Autodesk Inventor part; units mm, degrees
ref_plane "YZ Plane" through (0, 0, 0) normal (1, 0, 0) x (0, 1, 0)
ref_plane "XZ Plane" through (0, 0, 0) normal (0, 1, 0) x (-1, 0, 0)
ref_plane "XY Plane" through (0, 0, 0) normal (0, 0, 1) x (1, 0, 0)
sketch "Sketch_36" plane through (0, 0, 0) normal (0, 0, 1) x (1, 0, 0)
  line L0 (1.5, 0) -> (-1.5, 0)
  arc A0 (0, 1.6) -> (0.1, 1.5) centre (0.1, 1.6) ccw
  line L1 (0.1, 1.5) -> (2.9, 1.5)
  arc A1 (2.9, 1.5) -> (3, 1.6) centre (2.9, 1.6) ccw
  line L2 (3, 1.6) -> (3, 2.025)
  line L3 (3, 2.025) -> (1.6561, 2.025)
  arc A2 (1.3439, 2.025) -> (1.6561, 2.025) centre (1.5, 2.5) ccw
  line L4 (1.3439, 2.025) -> (0, 2.025)
  line L5 (0, 2.025) -> (0, 1.6)
revolve "Revolution1" add sketch "Sketch_36" angle 360 about axis through (1.5, 0, 0) along (1, 0, 0)
sketch "Sketch_37" plane through (0, 0, 0) normal (0, 0, 1) x (1, 0, 0)
  line L0 (1.5, 0) -> (-1.5, 0)
  line L1 (0, 3.175) -> (0, 1.925)
  line L2 (0, 1.925) -> (0.05, 1.925)
  arc A0 (0.05, 1.925) -> (0.15, 2.025) centre (0.05, 2.025) ccw
  line L3 (0.15, 2.025) -> (0.15, 3.075)
  line L4 (0.15, 3.075) -> (2.85, 3.075)
  line L5 (2.85, 3.075) -> (2.85, 2.025)
  arc A1 (2.85, 2.025) -> (2.95, 1.925) centre (2.95, 2.025) ccw
  line L6 (2.95, 1.925) -> (3, 1.925)
  line L7 (3, 1.925) -> (3, 3.175)
  line L8 (3, 3.175) -> (0, 3.175)
revolve "Revolution2" cut sketch "Sketch_37" angle 360 about axis through (1.5, 0, 0) along (1, 0, 0)
sketch "Sketch_38" plane through (0, 0, 0) normal (0, 0, 1) x (1, 0, 0)
  line L0 (50, 0) -> (-50, 0)
  line L1 (0.025, 3.175) -> (0.04, 2.8625)
  line L2 (0.04, 2.8625) -> (0.025, 2.55)
  line L3 (0.025, 2.55) -> (0.025, 1.925)
  line L4 (0.025, 1.925) -> (0.055, 1.925)
  line L5 (0.055, 1.925) -> (0.085, 2.55)
  line L6 (0.085, 2.55) -> (0.085, 2.8625)
  line L7 (0.085, 2.8625) -> (0.055, 3.175)
  line L8 (0.055, 3.175) -> (0.025, 3.175)
revolve "Revolution3" add sketch "Sketch_38" angle 360 about axis through (50, 0, 0) along (1, 0, 0)
sketch "Sketch_39" plane through (0, 0, 0) normal (0, 0, 1) x (1, 0, 0)
  line L0 (50, 0) -> (-50, 0)
  line L1 (2.915, 2.8625) -> (2.915, 2.55)
  line L2 (2.915, 2.55) -> (2.945, 1.925)
  line L3 (2.945, 1.925) -> (2.975, 1.925)
  line L4 (2.975, 1.925) -> (2.975, 2.55)
  line L5 (2.975, 2.55) -> (2.96, 2.8625)
  line L6 (2.96, 2.8625) -> (2.975, 3.175)
  line L7 (2.975, 3.175) -> (2.945, 3.175)
  line L8 (2.945, 3.175) -> (2.915, 2.8625)
revolve "Revolution4" add sketch "Sketch_39" angle 360 about axis through (50, 0, 0) along (1, 0, 0)
properties part number "W 638/3 R-2Z_PART1"
Here's how the part is built. I have some questions about the finished solid (model axes, mm). Give positions to 0.01 mm unless a question says otherwise; leave off trailing zeros. Write each loop counter-clockwise with the first axis right and the second up, starting at its lowest first coordinate (ties: lowest second). Pieces come first, ordered by that corner, then holes.
(1) Will these pins go through, and if not, where does the flat tip stop? pin 1 (3 mm diameter, centred on y = -1.5, z = -2.5, fed in from +X); pin 2 (1.5 mm diameter, centred on y = 0, z = 0.5, fed in from +X); pin 3 (1 mm diameter, centred on x = 1.5, y = 1, fed in from +Z).
Output values:
pin 1: stops at x = 3
pin 2: passes through
pin 3: stops at z = 1.96
(2) Imagine slicing it at A-A, the plane x = 0.95. Write out the boundary of the cut face in (y, z) (3 decimals), and give its area (3 significant figures).
Output values:
outline: circle Ø4.05 at (0, 0); hole circle Ø3 at (0, 0)
area: 5.81 mm2
(3) Thinking about a two-plate mould opening in Y: for faces 1 (the face through (2.245, -0.439, 1.977)), 2 (the face through (1.52, -1.5, 0.07)), which applies, pulls with the +Y half, pulls with the -Y half, needs draft (parallel to the pull), parting line crosses it, or undercut?
Output values:
face 1: parting line crosses it
face 2: undercut
(4) If I drill on L1, parallel to Z at x = 1, y = 0 (3 decimals); L2, parallel to Z at x = 1.75, y = 0.5; L3, parallel to Y at x = 0.45, z = 0.25, over which ranges is the centre line in solid material (lowest first)?
Output values:
L1: z = -2.025 to -1.5, 1.5 to 2.025
L2: z = -1.96 to -1.41, 1.41 to 1.96
L3: y = -2.01 to -1.48, 1.48 to 2.01
